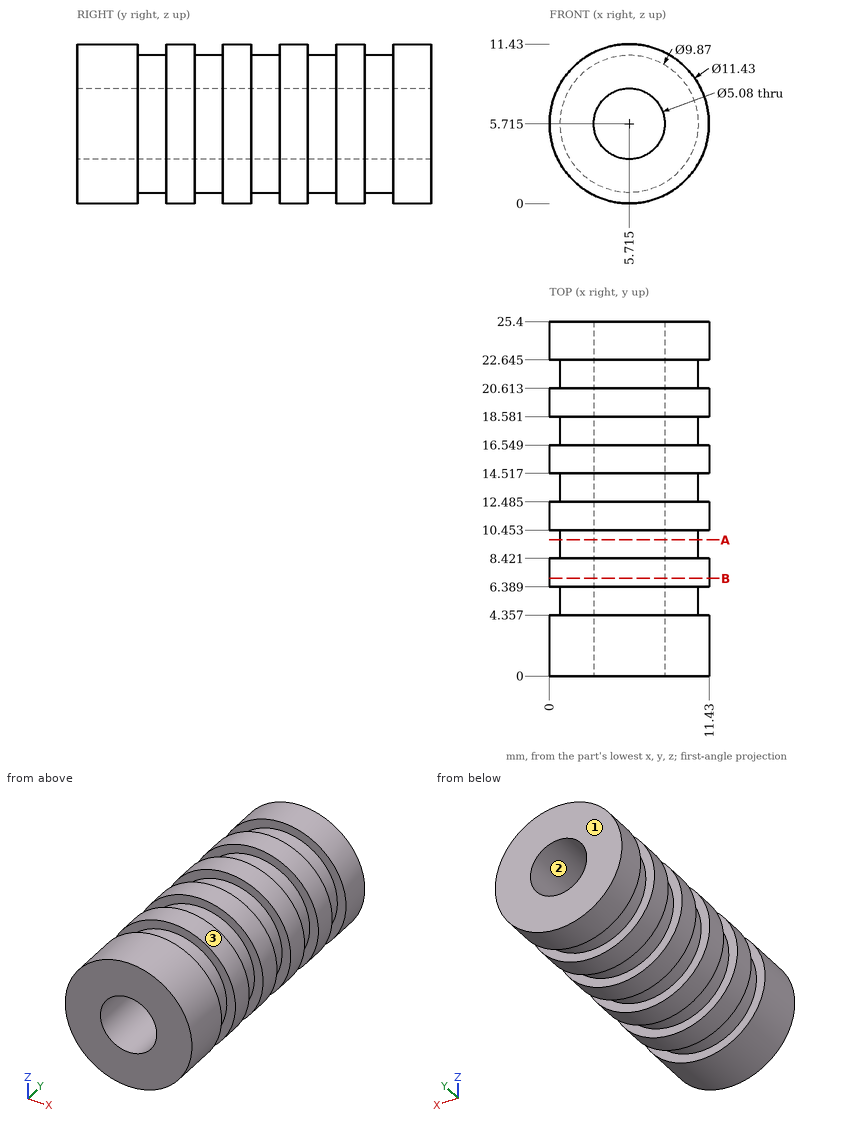
Check sheet for the drawn part. Datum: minimum x, y, z corner. Units: mm. Give positions to 0.01 mm unless a question says otherwise; leave off trailing zeros. Write each loop counter-clockwise with the first axis right and the second up, starting at its lowest first coordinate (ties: lowest second). Pieces come first, ordered by that corner, then holes. Notation, with made-up numbers: M -2.75,63 L 26.25,63 A14 ccw 26.25,71 Z; hole C 84,40 d5. An arc over 180 degrees is marked long. Write item = value, one per line.
(1) Draft check along X on the marked faces 1, 2 and 3. Enter one of: released by +X, released by -X, zero draft, split by the parting line, or undercut.
Found:
face_1 = zero draft
face_2 = undercut
face_3 = split by the parting line
(2) Sectioned sample at B-B (y = 7). Record the cut outline in (x, z) (1 decimal).
Found:
outline = C 5.7,5.7 d11.4; hole C 5.7,5.7 d5.1
(3) Go/stop test with flat-tipped pins: pin 1 Ø1.5 at (y, z) = (12, 1.5) entering from +X; pin 2 Ø5 at (x, y) = (9.5, 12.5) entering from +Z; pin 3 Ø1 at (x, y) = (7.5, 9) entering from +Z; pin 4 Ø3 at (x, z) = (5.715, 5.715) entering from +Y. Record where each tip stops, or that it passes through.
Found:
pin_1 = 10.26
pin_2 = 11.28
pin_3 = 10.48
pin_4 = through
(4) Material ranges on line 1 (Z direction, x = 7.25, y = 5) (1 decimal); line 2 (Z direction, x = 4, y = 9.5); line 3 (X direction, y = 11.25, z = 6.25) (1 decimal), recorded low to high.
Found:
line_1 = 1 to 3.7, 7.7 to 10.4
line_2 = 1.09 to 3.84, 7.59 to 10.34
line_3 = 0 to 3.2, 8.2 to 11.4
(5) Sectioned sample at A-A (y = 9.75). Record the cut outline in (x, z) (1 decimal).
Found:
outline = C 5.7,5.7 d9.9; hole C 5.7,5.7 d5.1
